```python
from build123d import *

# Parameters (mm, degrees)
SKETCH1_R               = 5
BOSS_EXTRUDE1_DEPTH     = 20
SKETCH2_W               = 10.491339254
SKETCH2_H               = 19.291026948
CUT_EXTRUDE1_DEPTH      = 17.60180745
CUT_EXTRUDE1_DEPTH_BACK = 17.60180745


with BuildPart() as part:
    # Sketch1 → Boss-Extrude1 (new body)
    with BuildSketch(Plane.XY):
        with BuildLine():
            Line((16.60180745, -10), (6.588404709, 4.537942638))
            ThreePointArc((6.588404709, 4.537942638), (0, 8), (-6.588404709, 4.537942638))
            Line((-6.588404709, 4.537942638), (-16.60180745, -10))
            Line((-16.60180745, -10), (16.60180745, -10))
        make_face()
        Circle(SKETCH1_R, mode=Mode.SUBTRACT)
    extrude(amount=BOSS_EXTRUDE1_DEPTH)

    # Sketch2 → Cut-Extrude1 (cut, two sides)
    with BuildSketch(Plane(origin=(0, 0, 0), x_dir=(0, 0, -1), z_dir=(1, 0, 0))) as cut_extrude1_sk:
        with Locations((-10, 2.276563947)):
            Rectangle(SKETCH2_W, SKETCH2_H)
    extrude(amount=CUT_EXTRUDE1_DEPTH, mode=Mode.SUBTRACT)
    extrude(cut_extrude1_sk.sketch, amount=-CUT_EXTRUDE1_DEPTH_BACK, mode=Mode.SUBTRACT)


solid = part.part
```
For this review, take the finished solid that the model builds, in its own axes (mm). A direction names the side the tool comes from. Round coordinates to 2 decimals unless told otherwise and drop trailing zeros. Write each loop counter-clockwise with the first axis right and the second up, starting at its lowest first coordinate (ties: lowest second). Pieces come first, ordered by that corner, then holes.
1) For line 1 along Z through (x, y) = (9, -4.75); line 2 along Y through (x, z) = (0, 18.35); line 3 along X through (y, z) = (0, 1.85), list the stretches that pass through material, from the lowest coordinate up.
Answer below:
line 1: z = 0 to 4.75, 15.25 to 20
line 2: y = -10 to -5, 5 to 8
line 3: x = -9.71 to -5, 5 to 9.71
2) Take a section at A-A on x = 0. Give the boundary of the cut face in (y, z), then the cut area to 3 significant figures.
Answer below:
outline: (-10, 0) - (-5, 0) - (-5, 4.75) - (-7.37, 4.75) - (-7.37, 15.25) - (-5, 15.25) - (-5, 20) - (-10, 20) - close; (5, 0) - (8, 0) - (8, 4.75) - (5, 4.75) - close; (5, 15.25) - (8, 15.25) - (8, 20) - (5, 20) - close
area: 104 mm2
3) Mouldability with a two-part tool opening along Y and no side actions: class faces 1 (the face through (3, -5, 15.246)), 2 (the face through (-1.08, -4.88, 17.59)), 3 (the face through (0, -7.369, 10)) as +Y half, -Y half, draft (parallel to the pull), parting line (faces both ways), or undercut.
Answer below:
face 1: draft
face 2: undercut
face 3: +Y half
4) Machinability: for faces 4 (the face through (3, -5, 4.754)), 5 (the face through (-15.975, -9.091, 9.86)), which of the approach directions +Z, -Z, +X, -X, +Y, -Y give a long, thin tool a straight path to every point of the face, cutting with its end or side? Answer none if there is none.
Answer below:
face 4: +X, -X, +Y
face 5: +Z, -Z, -X, +Y
5) Take a section at B-B on y = 6.5. Give the boundary of the cut face in (x, z), then the cut area to 3 significant figures.
Answer below:
outline: (-4.66, 0) - (4.66, 0) - (4.66, 4.75) - (-4.66, 4.75) - close; (-4.66, 15.25) - (4.66, 15.25) - (4.66, 20) - (-4.66, 20) - close
area: 88.7 mm2
6) Take a section at C-C on y = -2.5. Give the boundary of the cut face in (x, z).
Answer below:
outline: (-11.44, 0) - (-4.33, 0) - (-4.33, 4.75) - (-11.44, 4.75) - close; (-11.44, 15.25) - (-4.33, 15.25) - (-4.33, 20) - (-11.44, 20) - close; (4.33, 0) - (11.44, 0) - (11.44, 4.75) - (4.33, 4.75) - close; (4.33, 15.25) - (11.44, 15.25) - (11.44, 20) - (4.33, 20) - close
7) Insertion check: pin 1 Ø10 at (y, z) = (0.5, 16) entering from -X; pin 2 Ø3 at (y, z) = (-1, 15.5) entering from -X; pin 3 Ø1 at (y, z) = (4.5, 15.5) entering from +X. Each pin has a flat end and moves straight along its axis. Give the tip position at first contact, or say it passes through.
Answer below:
pin 1: stops at x = -12.81
pin 2: stops at x = -11.44
pin 3: stops at x = 6.96
8) Take a section at D-D on z = 18.75. Give the boundary of the cut face in (x, y).
Answer below:
outline: (-16.6, -10) - (16.6, -10) - (6.59, 4.54) arc R8 ccw to (-6.59, 4.54) - close; hole circle Ø10 at (0, 0)
